Source: CAD feature listing. Evaluate the final solid. Frame: model axes, mm. Face numbers are marked on the shaded views. A direction names the side the tool comes from. Coordinates: 2 decimals unless noted, no trailing zeros. Write each loop counter-clockwise with the first axis right and the second up, starting at its lowest first coordinate (ties: lowest second). Pieces come first, ordered by that corner, then holes. Notation, with made-up numbers: M 41.5,32.5 L 87.5,32.5 A17 ccw 87.5,42.5 Z; hole C 47.25,4 d6. An arc over 180 degrees is marked long. Answer as CSV lines item,"result". Start each with the question number.
1. Mould query, pull axis Y, two halves, no side actions, for the marked faces 1, 2, 3 and 4. Classes: pulls with the +Y half, pulls with the -Y half, needs draft (parallel to the pull), parting line crosses it, or undercut.
2. Section A-A on x = -10. Return the cut outline in (y, z).
3. Section C-C on y = -15. Return the cut outline in (x, z), plus the area to 3 significant figures.
4. Contact query for flat-ended pins moving along their axis: pin 1 Ø6 at (x, y) = (-10, 0) entering from +Z; pin 2 Ø7 at (y, z) = (0, 11.5) entering from -X; pin 3 Ø9.5 at (x, z) = (32, 12.5) entering from -Y. Output: stop coordinate, or through.
5. Reachability of the marked faces 5, 6, 7, 8 and 9 from +Z, -Z, +X, -X, +Y, -Y: full face, straight path, thin tool, end or side. Return the list, or none.
6. Line query: probe 1 along X at (y, z) = (0, 11.5) (3 decimals); probe 2 along Y at (x, z) = (-30, 4.15); probe 3 along Y at (x, z) = (38.5, 14.25) (3 decimals). Output: solid intervals per line, ascending. Write a range as [from, to].
7. Section D-D on z = 6. Return the cut outline in (x, y).
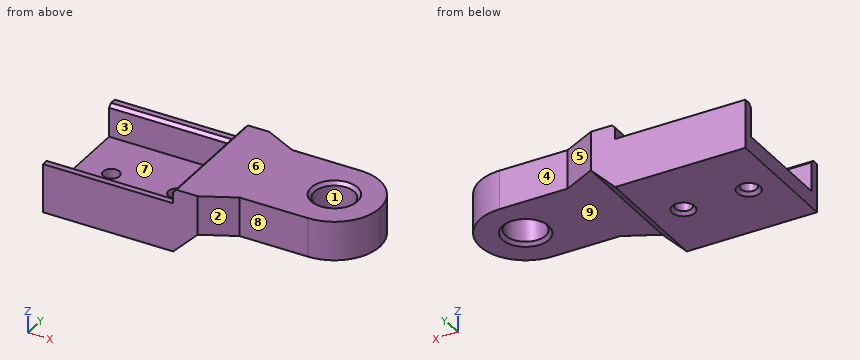
Solid Edge part; units mm, degrees
sketch "Sketch1" plane through (0, 0, 0) normal (0, -1, 0) x (1, 0, 0)
  line L0 (-40, 15) -> (-40, 0)
  line L1 (-40, 0) -> (0, 0)
  line L2 (0, 0) -> (7.5, 7.5)
  line L3 (7.5, 7.5) -> (52.5, 7.5)
  line L4 (52.5, 7.5) -> (52.5, 19.5)
  line L5 (52.5, 19.5) -> (0, 19.5)
  line L6 (0, 19.5) -> (0, 15)
  line L7 (0, 15) -> (-40, 15)
  dimension "D1" = 40
  dimension "D2" = 52.5
  dimension "D3" = 7.5
extrude "Protrusion1" add sketch "Sketch1" along normal mid plane 38
sketch "Sketch2" plane through (-10, -18, 15) normal (0, 0, 1) x (1, 0, 0)
  line L0 (10, 34.1) -> (-30, 34.1)
  line L1 (-30, 34.1) -> (-30, 1.9)
  line L2 (-30, 1.9) -> (10, 1.9)
  line L3 (10, 1.9) -> (10, 34.1)
  dimension "D1" = 10
extrude "ExtrudedCutout_1" cut sketch "Sketch2" against normal blind 10
sketch "Sketch3" plane through (25, 0, 7.5) normal (0, 0, -1) x (1, 0, 0)
  line L0 (-17.5, 19) -> (-7.5, 14)
  line L1 (-7.5, 14) -> (27.5, 14)
  line L2 (27.5, 14) -> (27.5, -14)
  line L3 (27.5, -14) -> (-7.5, -14)
  line L4 (-7.5, -14) -> (-17.5, -19)
  dimension "D1" = 17.5
  dimension "D2" = 17.5
extrude "ExtrudedCutout_2" cut sketch "Sketch3" against normal blind 41 material side at (12.5224, -16.5447, 7.5)
fillet "Round1" radius 14 2 edges at (52.5, 14, 13.5) (52.5, -14, 13.5)
hole "Hole_1" at (38.5, 0, 7.5) direction (0, 0, 1) diameter 12.25 end up to next
hole "Hole_2" at (-10, 0, 5) direction (0, 0, -1) diameter 5 end up to next
hole "Hole1" at (-30, 0, 5) direction (0, 0, -1) diameter 5 end up to next
chamfer "Chamfer1" distance 1 angle 45 4 edges at (38.5, -6.125, 7.5) (44.625, 0, 19.5) (-12.5, 0, 0) (-32.5, 0, 0)
chamfer "Chamfer_2" distance 1 angle 45 3 edges at (-20, 16.1, 15) (-20, -16.1, 15) (0, 0, 19.5)
properties material "Polyethylene, low density"
Values:
1,face 1,"undercut"
1,face 2,"pulls with the -Y half"
1,face 3,"undercut"
1,face 4,"pulls with the +Y half"
2,outline,"M -19,0 L -3.5,0 L -2.5,1 L -2.5,5 L -16.1,5 L -16.1,14 L -17.1,15 L -19,15 Z; M 2.5,1 L 3.5,0 L 19,0 L 19,15 L 17.1,15 L 16.1,14 L 16.1,5 L 2.5,5 Z"
3,outline,"M -40,0 L 0,0 L 7.5,7.5 L 15.5,7.5 L 15.5,19.5 L 1,19.5 L 0,18.5 L 0,5 L -40,5 Z"
3,area,"414 mm²"
4,pin 1,"z = 5"
4,pin 2,"x = 0"
4,pin 3,"y = -14"
5,face 5,"+Z, -Z, +X, +Y"
5,face 6,"+Z, +X, -X, +Y, -Y"
5,face 7,"+Z, -X"
5,face 8,"+Z, -Z, +X, -Y"
5,face 9,"-Z, +X, +Y, -Y"
6,probe 1,"[0, 32.375], [44.625, 52.5]"
6,probe 2,"[-19, -2.5], [2.5, 19]"
6,probe 3,"[-14, -6.125], [6.125, 14]"
7,outline,"M -40,-19 L 6,-19 L 6,19 L -40,19 L -40,16.1 L 0,16.1 L 0,-16.1 L -40,-16.1 Z"
